Design review of the part built by this model. Coordinates are the model's own, in mm. Face numbers are marked on the shaded views. A direction names the side the tool comes from. Round coordinates to 2 decimals unless told otherwise and drop trailing zeros. Order: outer loops, then holes, each group sorted by start corner. A loop starts at its lowest first (then second) coordinate and runs counter-clockwise, first axis right, second up. Notation, with made-up numbers: (3, -12) - (14, -12) arc R15 cw to (14, 0) - close; hole circle Ø4 at (-24.75, 33.5). An arc over 180 degrees is marked (long way). Write item = value, one per line.
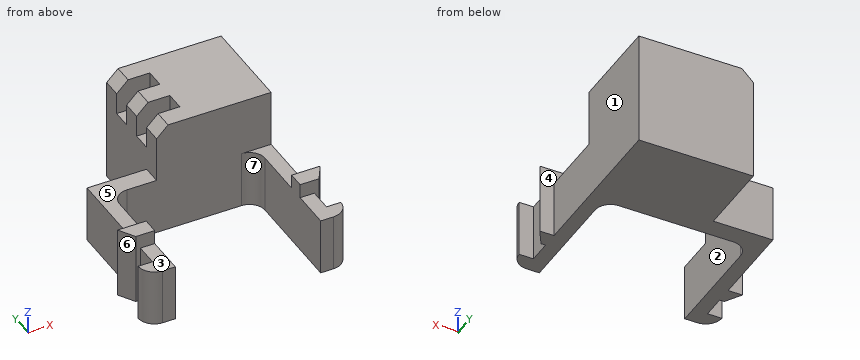
from build123d import *

# Parameters (mm, degrees)
PAD017_DEPTH           = 5
PAD020_DEPTH           = 6.25
SKETCH038_W            = 10
SKETCH038_H            = 1.65
PAD021_DEPTH           = 5
SKETCH089_W            = 10
SKETCH089_H            = 1.65
PAD058_DEPTH           = 10
SKETCH086_W            = 10
SKETCH086_H            = 1.65
PAD059_DEPTH           = 7.1
SKETCH087_W            = 7.1
SKETCH087_H            = 1.65
PAD060_DEPTH           = 10
SKETCH088_W            = 10
SKETCH088_H            = 1.65
PAD061_DEPTH           = 10
LINEARPATTERN020_COUNT = 2
LINEARPATTERN020_PITCH = 3.3
CHAMFER010_SIZE        = 1


with BuildPart() as obj1:
    # Sketch034 → Pad017 (new body)
    with BuildSketch(Plane.XY):
        with BuildLine():
            Line((-1.35, -1.8), (-1.35, 6))
            ThreePointArc((0, 7.35), (-0.954594, 6.954594), (-1.35, 6))
            Line((0, 9), (0, 7.35))
            Line((-2.6, 9), (0, 9))
            Line((-2.6, -1.8), (-2.6, 9))
            Line((-3.85, -1.8), (-2.6, -1.8))
            ThreePointArc((-3.85, -1.8), (-3.439949, -2.789949), (-2.45, -3.2))
            Line((-1.35, -3.2), (-2.45, -3.2))
            Line((-1.35, -1.8), (-1.35, -3.2))
        make_face()
    extrude(amount=PAD017_DEPTH)

    # Sketch037 → Pad020 (join)
    with BuildSketch(Plane.XY):
        Polygon((-1.35, 0.2), (-1.35, 1.6), (-2.6, 1.6), (-3.85, 1.6), (-3, 0.2), (-2.6, 0.2), align=None)
    extrude(amount=PAD020_DEPTH)


with BuildPart() as body031:
    # Mirror002: instance of _obj1
    add(obj1.part.mirror(Plane(origin=(5, 0, 0), x_dir=(0, 1, 0), z_dir=(-1, 0, 0))))

    # Fusion002: union _obj1
    add(obj1.part)


with BuildPart() as body031_1:
    # Clone003 placement: moved
    add(body031.part.moved(Location((-5, 0, 0))))

    # Sketch038 → Pad021 (new body)
    with BuildSketch(Plane.XY):
        with Locations((0, 8.175)):
            Rectangle(SKETCH038_W, SKETCH038_H)
    extrude(amount=PAD021_DEPTH)

    # Sketch089 → Pad058 (new body)
    with BuildSketch(Plane.XY):
        with Locations((2.6, 8.175)):
            Rectangle(SKETCH089_W, SKETCH089_H)
    extrude(amount=PAD058_DEPTH)

    # Sketch086 → Pad059 (join)
    with BuildSketch(Plane.XY):
        with Locations((2.6, 9.825)):
            Rectangle(SKETCH086_W, SKETCH086_H)
    pad059 = extrude(amount=PAD059_DEPTH)

    # Sketch087 → Pad060 (join)
    with BuildSketch(Plane.XY):
        with Locations((4.05, 9.825)):
            Rectangle(SKETCH087_W, SKETCH087_H)
    pad060 = extrude(amount=PAD060_DEPTH)

    # Sketch088 → Pad061 (join)
    with BuildSketch(Plane.XY):
        with Locations((2.6, 11.475)):
            Rectangle(SKETCH088_W, SKETCH088_H)
    pad061 = extrude(amount=PAD061_DEPTH)

    # LinearPattern020: Pad061, Pad060, Pad059 ×2
    with Locations(*[(0, i * LINEARPATTERN020_PITCH, 0) for i in range(1, LINEARPATTERN020_COUNT)]):
        add(pad061)
        add(pad060)
        add(pad059)

    # Chamfer010
    chamfer010_edges = [body031_1.edges().sort_by_distance(p)[0] for p in [
        (-2.4, 14.775, 10),
        (-2.4, 11.475, 10),
        (-2.4, 8.175, 10),
    ]]
    chamfer(chamfer010_edges, length=CHAMFER010_SIZE)


with BuildPart() as body031_2:
    # Body031 placement: moved
    add(body031_1.part.moved(Location((-5, 0, 0))))


solid = body031_2.part
1) Clearance check with flat-ended pins moving along their axes: pin 1 Ø5 at (x, y) = (-2.5, 3.5) entering from +Z; pin 2 Ø2 at (x, z) = (-12.5, 2.5) entering from +Y; pin 3 Ø1.9 at (y, z) = (2, 2.5) entering from -X; pin 4 Ø5 at (y, z) = (8.5, 6.5) entering from +X. State where each tip first meets the part, or that it passes through.
Findings:
pin_1 = through
pin_2 = 9
pin_3 = -13.85
pin_4 = 2.6
2) To check wall thickness, follow L1, parallel to Y at x = -4, z = 6.75; L2, parallel to X at y = 13.75, z = 6.25; L3, parallel to Y at x = -9.5, z = 3. State the ranges of each line that lie inside material, in increasing order. Write a range as from..to.
Findings:
L1 = 7.35..15.6
L2 = -7.4..2.6
L3 = 7.35..9
3) We need section B-B on z = 5.25. Write out the cut boundary in (x, y), and give its area (3 significant figures).
Findings:
outline = (-13.85, 1.6) - (-13, 0.2) - (-11.35, 0.2) - (-11.35, 1.6) - close; (-7.4, 7.35) - (2.6, 7.35) - (2.6, 15.6) - (-7.4, 15.6) - close; (1.35, 0.2) - (3, 0.2) - (3.85, 1.6) - (1.35, 1.6) - close
area = 88.3 mm^2
4) For the marked faces 1, 2, 3 and 4, list the 3-axis set-ups (+Z, -Z, +X, -X, +Y, -Y) from which the entire face can be reached by the end or side of a thin tool; tool diameter is ignored.
Findings:
face_1 = +Z, -Z, +X, +Y
face_2 = +Z, -Z, -Y
face_3 = +Z, +X, -X, -Y
face_4 = +Z, +X
5) We need section C-C on x = -5. Write out the cut boundary in (y, z).
Findings:
outline = (7.35, 0) - (15.6, 0) - (15.6, 10) - (13.95, 10) - (13.95, 7.1) - (12.3, 7.1) - (12.3, 10) - (10.65, 10) - (10.65, 7.1) - (9, 7.1) - (9, 10) - (7.35, 10) - close
6) The part is to be moulded in two halves that separate along Y. For the marked faces 5, 6 and 7, say which applies: released by +Y, released by -Y, zero draft, split by the parting line, or undercut.
Findings:
face_5 = zero draft
face_6 = undercut
face_7 = released by -Y
7) We need section D-D on z = 9.5. Write out the cut boundary in (x, y), and give its area (3 significant figures).
Findings:
outline = (-6.9, 7.35) - (2.6, 7.35) - (2.6, 15.6) - (-6.9, 15.6) - (-6.9, 13.95) - (-4.5, 13.95) - (-4.5, 12.3) - (-6.9, 12.3) - (-6.9, 10.65) - (-4.5, 10.65) - (-4.5, 9) - (-6.9, 9) - close
area = 70.5 mm^2
8) We need section A-A on y = 4. Write out the cut boundary in (x, z), and give its area (3 significant figures).
Findings:
outline = (-12.6, 0) - (-11.35, 0) - (-11.35, 5) - (-12.6, 5) - close; (1.35, 0) - (2.6, 0) - (2.6, 5) - (1.35, 5) - close
area = 12.5 mm^2
